Could you check a few things on this model? Use its own coordinates, in mm. Coordinates: 2 decimals unless noted, no trailing zeros. Loops run counter-clockwise (first coordinate to the right, second up) from the corner with the lowest first, then second, coordinate; pieces in that order, holes last.
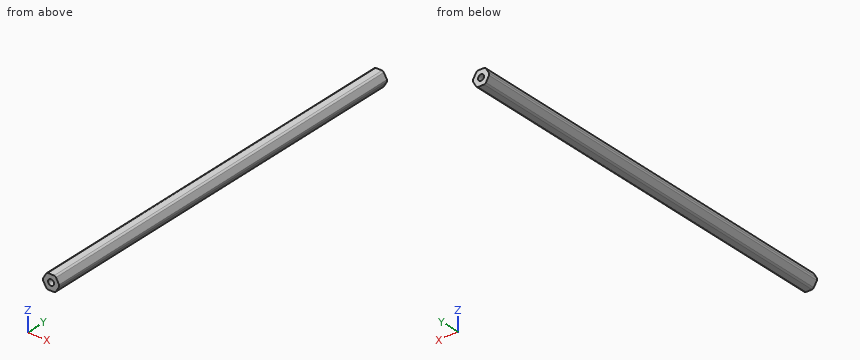
Autodesk Inventor part; units mm, degrees
ref_plane "YZ Plane" through (0, 0, 0) normal (1, 0, 0) x (0, 1, 0)
ref_plane "XZ Plane" through (0, 0, 0) normal (0, 1, 0) x (-1, 0, 0)
ref_plane "XY Plane" through (0, 0, 0) normal (0, 0, 1) x (1, 0, 0)
sketch "Sketch1" plane through (0, 0, 0) normal (0, 1, 0) x (-1, 0, 0)
  line L0 (7.3323, 0) -> (3.6662, -6.35)
  line L1 (3.6662, -6.35) -> (-3.6662, -6.35)
  line L2 (-3.6662, -6.35) -> (-7.3323, 0)
  line L3 (-7.3323, 0) -> (-3.6662, 6.35)
  line L4 (-3.6662, 6.35) -> (3.6662, 6.35)
  line L5 (3.6662, 6.35) -> (7.3323, 0)
  circle A0 centre (0, 0) radius 2.5527
  circle A1 centre (0, 0) radius 6.8758
  point P0 (2.637, -6.35)
  point P1 (4.1808, -5.4587)
  point P2 (6.8178, -0.8913)
  point P3 (6.8178, 0.8913)
  point P4 (4.1808, 5.4587)
  point P5 (2.637, 6.35)
  point P6 (-2.637, 6.35)
  point P7 (-4.1808, 5.4587)
  point P8 (-6.8178, 0.8913)
  point P9 (-6.8178, -0.8913)
  point P10 (-4.1808, -5.4587)
  point P11 (-2.637, -6.35)
  dimension "d0" = 6.35
  dimension "d1" = 5.1054
  dimension "d2" = 13.7516
extrude "Extrusion1" add sketch "Sketch1" along normal blind 317.5 contours L0 A1 L1 L2 L3 L4 L5
move faces "Move1" translate (0, 12.7, 0) faces at (-0.1026, 317.5, -5.078)
move faces "Move2" translate (0, -12.7, 0) faces at (-0.1026, 0, -5.078)
properties part number "thunder hex 13in"
(1) Imagine slicing it at A-A, the plane x = 0. Write out the boundary of the cut face in (y, z), and give its area (3 significant figures).
Answers:
outline: (-12.7, -6.35) - (330.2, -6.35) - (330.2, -2.55) - (-12.7, -2.55) - close; (-12.7, 2.55) - (330.2, 2.55) - (330.2, 6.35) - (-12.7, 6.35) - close
area: 2,600 mm2
(2) I need wall thicknesses on probe 1 along Z at (x, y) = (0.5, 295); probe 2 along X at (y, z) = (97.5, 0); probe 3 along Z at (x, y) = (0, 114). Which ranges of each line are inside material? Lowest first, please.
Answers:
probe 1: z = -6.35 to -2.5, 2.5 to 6.35
probe 2: x = -6.88 to -2.55, 2.55 to 6.88
probe 3: z = -6.35 to -2.55, 2.55 to 6.35
(3) Imagine slicing it at B-B, the plane y = 34. Write out the boundary of the cut face in (x, z), and give its area (3 significant figures).
Answers:
outline: (-6.82, -0.89) - (-4.18, -5.46) arc R6.88 ccw to (-2.64, -6.35) - (2.64, -6.35) arc R6.88 ccw to (4.18, -5.46) - (6.82, -0.89) arc R6.88 ccw to (6.82, 0.89) - (4.18, 5.46) arc R6.88 ccw to (2.64, 6.35) - (-2.64, 6.35) arc R6.88 ccw to (-4.18, 5.46) - (-6.82, 0.89) arc R6.88 ccw to start; hole circle Ø5.11 at (0, 0)
area: 117 mm2
(4) For pin 1 (5 mm diameter, centred on y = 202.5, z = 4, fed in from -X); pin 2 (2 mm diameter, centred on x = -4.5, y = 278.5, fed in from -Z); pin 3 (6 mm diameter, centred on y = 69.5, z = 3.5, fed in from +X), each with a flat end and sliding along its axis, tell me the tip position at first contact or that it passes through.
Answers:
pin 1: stops at x = -6.47
pin 2: stops at z = -5.92
pin 3: stops at x = 6.86
